For this review, take the finished solid that the model builds, in its own axes (mm). A direction names the side the tool comes from. Round coordinates to 2 decimals unless told otherwise and drop trailing zeros. Write each loop counter-clockwise with the first axis right and the second up, starting at its lowest first coordinate (ties: lowest second). Pieces come first, ordered by that corner, then holes.
from build123d import *

# Parameters (mm, degrees)
EXTRUDE_1_DEPTH          = 61
SKETCH_3_W               = 5
SKETCH_3_H               = 62
EXTRUDE_2_DEPTH          = 57
CUT_EXTRUDE_11_DEPTH     = 10
SKETCH_16_R              = 7.5
SKETCH_16_R_2            = 1.25
CUT_EXTRUDE_12_DEPTH     = 10
PATTERN_CIRCULAR_7_COUNT = 6
CUT_EXTRUDE_13_DEPTH     = 10
FILLET_2_R               = 10
SKETCH_18_R              = 12.5
SKETCH_18_R_2            = 1.25
CUT_EXTRUDE_14_DEPTH     = 10
PATTERN_CIRCULAR_8_COUNT = 4


with BuildPart() as part:
    # 草图1 → 凸台-拉伸1 (new body)
    with BuildSketch(Plane.XY):
        Polygon((0, 0), (57, 0), (57, -5), (5, -5), (5, -67), (0, -67), (0, -10.157289975), align=None)
    extrude(amount=EXTRUDE_1_DEPTH)

    # 草图3 → 凸台-拉伸2 (add)
    with BuildSketch(Plane.ZY):
        with Locations((2.5, 31)):
            Rectangle(SKETCH_3_W, SKETCH_3_H)
    extrude(amount=-EXTRUDE_2_DEPTH)

    # 草图15 → 切除-拉伸11 (cut)
    with BuildSketch(Plane(origin=(0, 0, 0), x_dir=(-1, 0, 0), z_dir=(0, 0, -1))):
        with BuildLine():
            ThreePointArc((-57, 33.5), (-48.652543264, 53.652543264), (-28.5, 62))
            Line((-28.5, 62), (-57, 62))
            Line((-57, 62), (-57, 33.5))
        make_face()
        with BuildLine():
            Line((0, 33.5), (0, 62))
            Line((0, 62), (-28.5, 62))
            ThreePointArc((-28.5, 62), (-8.347456736, 53.652543264), (0, 33.5))
        make_face()
    extrude(amount=-CUT_EXTRUDE_11_DEPTH, mode=Mode.SUBTRACT)

    # 草图16 → 切除-拉伸12 (cut)
    with BuildSketch(Plane(origin=(0, 0, 0), x_dir=(-1, 0, 0), z_dir=(0, 0, -1))):
        with Locations((-28.5, 33.5)):
            Circle(SKETCH_16_R)
        with Locations((-15, 33.5)):
            Circle(SKETCH_16_R_2)
    cut_extrude_12 = extrude(amount=-CUT_EXTRUDE_12_DEPTH, mode=Mode.SUBTRACT)

    # 阵列(圆周)7: 切除-拉伸12 ×6 about axis
    pattern_circular_7_axis = Axis((28.5, 33.5, 0), (0, 0, 1))
    for i in range(1, PATTERN_CIRCULAR_7_COUNT):
        add(cut_extrude_12.rotate(pattern_circular_7_axis, i * 360 / PATTERN_CIRCULAR_7_COUNT), mode=Mode.SUBTRACT)

    # 草图17 → 切除-拉伸13 (cut)
    with BuildSketch(Plane(origin=(5, 0, 0), x_dir=(0, 0, -1), z_dir=(1, 0, 0))):
        with BuildLine():
            Line((-61, -38.5), (-61, -67))
            Line((-61, -67), (-32.5, -67))
            ThreePointArc((-32.5, -67), (-52.652543264, -58.652543264), (-61, -38.5))
        make_face()
    extrude(amount=-CUT_EXTRUDE_13_DEPTH, mode=Mode.SUBTRACT)

    # 圆角2
    fillet_2_edges = [part.edges().sort_by_distance(p)[0] for p in [
        (57, -2.5, 61),
        (2.5, -67, 0),
    ]]
    fillet(fillet_2_edges, radius=FILLET_2_R)

    # 草图18 → 切除-拉伸14 (cut)
    with BuildSketch(Plane(origin=(5, 0, 0), x_dir=(0, 0, -1), z_dir=(1, 0, 0))):
        with Locations(Location((-32.5, -38.5, 0), (0, 0, 90))):
            Circle(SKETCH_18_R)
        with Locations(Location((-45.935028843, -51.935028843, 0), (0, 0, 90))):
            Circle(SKETCH_18_R_2)
    cut_extrude_14 = extrude(amount=-CUT_EXTRUDE_14_DEPTH, mode=Mode.SUBTRACT)

    # 阵列(圆周)8: 切除-拉伸14 ×4 about axis
    pattern_circular_8_axis = Axis((0, -38.5, 32.5), (1, 0, 0))
    for i in range(1, PATTERN_CIRCULAR_8_COUNT):
        add(cut_extrude_14.rotate(pattern_circular_8_axis, i * 360 / PATTERN_CIRCULAR_8_COUNT), mode=Mode.SUBTRACT)


solid = part.part
(1) Mouldability with a two-part tool opening along X and no side actions: class faces 1 (the face through (40.75, 33.45, 2.46)), 2 (the face through (28, 24, 5)), 3 (the face through (21.59, 20.57, 2.46)), 4 (the face through (0, -27, 23)) as pulls with the +X half, pulls with the -X half, needs draft (parallel to the pull), parting line crosses it, or undercut.
Geometry check:
face 1: undercut
face 2: needs draft
face 3: undercut
face 4: pulls with the -X half
(2) For faces 5 (the face through (31, -5, 30)), 6 (the face through (34.095, 21.33, 2.465)), list the 3-axis set-ups (+Z, -Z, +X, -X, +Y, -Y) from which the entire face can be reached by the end or side of a thin tool; tool diameter is ignored.
Geometry check:
face 5: +Z, -Z, +X, -Y
face 6: +Z, -Z
(3) For line 1 along Y through (x, z) = (35, 4); line 2 along Y through (x, z) = (30.5, 22); line 3 along Z through (x, y) = (5.5, 44.5), list the stretches that pass through material, from the lowest coordinate up.
Geometry check:
line 1: y = -5 to 20.58, 23.03 to 29.76, 37.24 to 43.97, 46.42 to 61.25
line 2: y = -5 to 0
line 3: z = 0 to 5
(4) We need section D-D, the plane z = 15. Give the boundary of the cut face in (x, y).
Geometry check:
outline: (0, -67) - (5, -67) - (5, -5) - (57, -5) - (57, 0) - (0, 0) - close
(5) For pin 1 Ø3 at (x, y) = (21.75, 45.19) entering from +Z; pin 2 Ø15.5 at (x, z) = (32.5, 24) entering from -Y; pin 3 Ø17 at (x, z) = (21, 38.5) entering from +Y, all flat-tipped, find the tip position at first contact; note any pin that passes through.
Geometry check:
pin 1: stops at z = 5
pin 2: stops at y = -5
pin 3: stops at y = 0
(6) We need section A-A, the plane z = 27. Give the boundary of the cut face in (x, y), and give its area (3 significant figures).
Geometry check:
outline: (0, -67) - (5, -67) - (5, -49.72) - (0, -49.72) - close; (0, -27.28) - (5, -27.28) - (5, -5) - (57, -5) - (57, 0) - (0, 0) - close
area: 483 mm2
(7) We need section B-B, the plane y = -40.5. Give the boundary of the cut face in (x, z), and give its area (3 significant figures).
Geometry check:
outline: (0, 0) - (5, 0) - (5, 20.16) - (0, 20.16) - close; (0, 44.84) - (5, 44.84) - (5, 60.93) - (0, 60.93) - close
area: 181 mm2
(8) We need section C-C, the plane x = 30. Give the boundary of the cut face in (y, z), and give its area (3 significant figures).
Geometry check:
outline: (-5, 0) - (26.15, 0) - (26.15, 5) - (0, 5) - (0, 61) - (-5, 61) - close; (40.85, 0) - (61.96, 0) - (61.96, 5) - (40.85, 5) - close
area: 541 mm2
